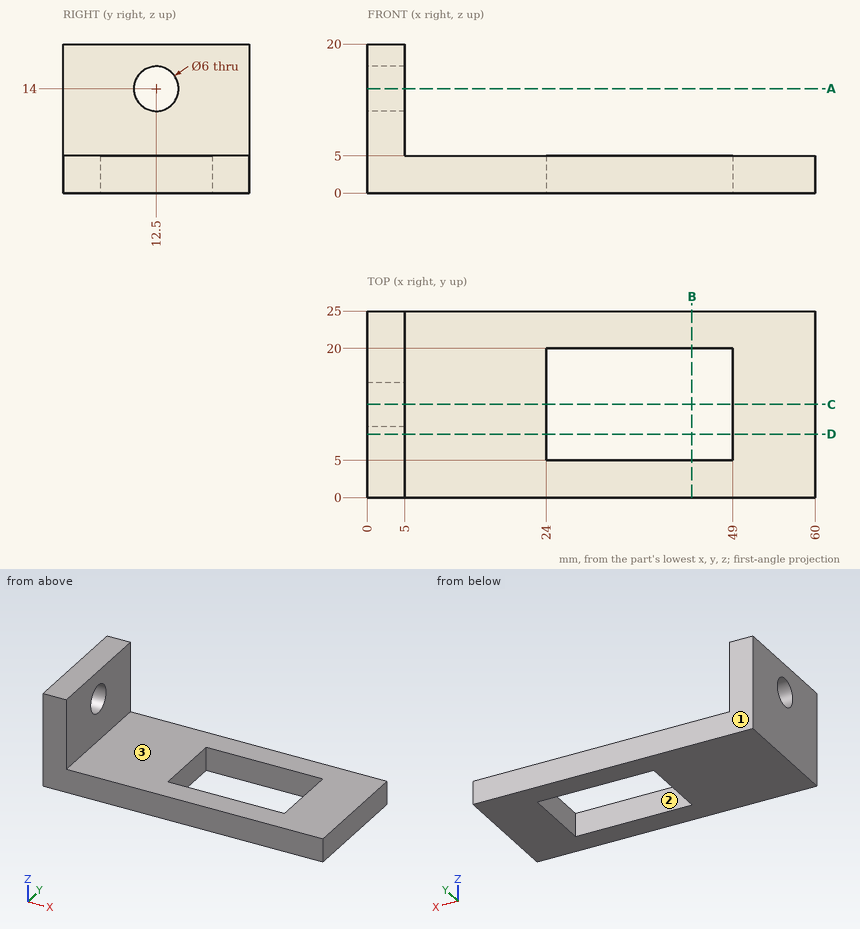
For this review, use the dimensioned drawing (mm, ordinates from the lowest corner) and the shaded views. A direction names the side the tool comes from. Give positions to 0.01 mm unless a question says otherwise; leave off trailing zeros. Order: outer loops, then holes, each group sorted by start corner. A loop starts at its lowest first (then second) coordinate and runs counter-clockwise, first axis right, second up.
1) Insertion check: pin 1 (7.5 mm diameter, centred on y = 9.5, z = 13, fed in from +X); pin 2 (12.5 mm diameter, centred on x = 22, y = 9, fed in from +Z). Each pin has a flat end and moves straight along its axis. Give the tip position at first contact, or say it passes through.
2) Take a section at C-C (y = 12.5). Give the boundary of the cut face in (x, z), then the cut area to 3 significant figures.
3) Take a section at D-D (y = 8.5). Give the boundary of the cut face in (x, z).
4) Take a section at B-B (x = 43.5). Give the boundary of the cut face in (y, z).
5) Take a section at A-A (z = 14). Give the boundary of the cut face in (x, y), then the cut area to 3 significant figures.
6) Wall thickness on line 1 (Z direction, x = 3.75, y = 12.5); line 2 (Y direction, x = 37, z = 3.5); line 3 (X direction, y = 10.75, z = 4): over which ranges is each line inside the solid? List them lowest first.
7) For the marked faces 1, 2 and 3, list the 3-axis set-ups (+Z, -Z, +X, -X, +Y, -Y) from which the entire face can be reached by the end or side of a thin tool; tool diameter is ignored.
Derived:
1. pin 1: stops at x = 5
1. pin 2: stops at z = 5
2. outline: (0, 0) - (24, 0) - (24, 5) - (5, 5) - (5, 11) - (0, 11) - close; (0, 17) - (5, 17) - (5, 20) - (0, 20) - close; (49, 0) - (60, 0) - (60, 5) - (49, 5) - close
2. area: 220 mm2
3. outline: (0, 0) - (24, 0) - (24, 5) - (5, 5) - (5, 20) - (0, 20) - close; (49, 0) - (60, 0) - (60, 5) - (49, 5) - close
4. outline: (0, 0) - (5, 0) - (5, 5) - (0, 5) - close; (20, 0) - (25, 0) - (25, 5) - (20, 5) - close
5. outline: (0, 0) - (5, 0) - (5, 9.5) - (0, 9.5) - close; (0, 15.5) - (5, 15.5) - (5, 25) - (0, 25) - close
5. area: 95.0 mm2
6. line 1: z = 0 to 11, 17 to 20
6. line 2: y = 0 to 5, 20 to 25
6. line 3: x = 0 to 24, 49 to 60
7. face 1: +Z, -Z, +X, -X, +Y
7. face 2: +Z, -Z
7. face 3: +Z, +X, +Y, -Y
